```python
from build123d import *

# Parameters (mm, degrees)
SKETCH002_R           = 15
SKETCH002_R_2         = 13.55
PAD002_DEPTH          = 3
PAD002_DEPTH_BACK     = 1.4
CHAMFER001_SIZE       = 1
CHAMFER002_SIZE       = 0.6
SKETCH003_R           = 13.55
PAD003_DEPTH          = 1
SKETCH004_W           = 1.1
SKETCH004_H           = 2.4
POCKET_DEPTH          = 0.8
SKETCH005_R           = 13.55
SKETCH005_R_2         = 12
PAD005_DEPTH          = 2
PAD006_DEPTH          = 2
POLARPATTERN001_COUNT = 4
SKETCH007_R           = 9.5
POCKET001_DEPTH       = 0.6
SKETCH008_R           = 1.3
POCKET002_DEPTH       = 7


with BuildPart() as part:
    # Sketch002 → Pad002 (new body, two sides)
    with BuildSketch(Plane.XY) as pad002_sk:
        Circle(SKETCH002_R)
        Circle(SKETCH002_R_2, mode=Mode.SUBTRACT)
    extrude(amount=-PAD002_DEPTH)
    extrude(pad002_sk.sketch, amount=PAD002_DEPTH_BACK)

    # Chamfer001
    chamfer001_edges = [part.edges().sort_by_distance(p)[0] for p in [
        (-15, 0, 1.4),
    ]]
    chamfer(chamfer001_edges, length=CHAMFER001_SIZE)

    # Chamfer002
    chamfer002_edges = [part.edges().sort_by_distance(p)[0] for p in [
        (-15, 0, -3),
    ]]
    chamfer(chamfer002_edges, length=CHAMFER002_SIZE)

    # Sketch003 → Pad003 (join)
    with BuildSketch(Plane.XY.offset(-3)):
        Circle(SKETCH003_R)
    extrude(amount=PAD003_DEPTH)

    # Sketch004 → Pocket (cut)
    with BuildSketch(Plane.XY):
        with Locations((13.5, 0)):
            Rectangle(SKETCH004_W, SKETCH004_H)
    pocket = extrude(amount=POCKET_DEPTH, mode=Mode.SUBTRACT)

    # Sketch005 → Pad005 (join)
    with BuildSketch(Plane.XY):
        Circle(SKETCH005_R)
        Circle(SKETCH005_R_2, mode=Mode.SUBTRACT)
    extrude(amount=-PAD005_DEPTH)

    # Sketch006 → Pad006 (join)
    with BuildSketch(Plane.XY):
        with BuildLine():
            ThreePointArc((12.310097, -2.170602), (12.5, 0), (12.310097, 2.170602))
            Line((7.878462, 1.389185), (12.310097, 2.170602))
            ThreePointArc((7.878462, -1.389185), (8, 0), (7.878462, 1.389185))
            Line((7.878462, -1.389185), (12.310097, -2.170602))
        make_face()
    pad006 = extrude(amount=-PAD006_DEPTH)

    # PolarPattern001: Pocket, Pad006 ×4 about axis
    polarpattern001_axis = Axis((0, 0, 0), (0, 0, 1))
    for i in range(1, POLARPATTERN001_COUNT):
        add(pocket.rotate(polarpattern001_axis, i * 360 / POLARPATTERN001_COUNT), mode=Mode.SUBTRACT)
        add(pad006.rotate(polarpattern001_axis, i * 360 / POLARPATTERN001_COUNT))

    # Sketch007 → Pocket001 (cut)
    with BuildSketch(Plane.XY):
        Circle(SKETCH007_R)
    extrude(amount=-POCKET001_DEPTH, mode=Mode.SUBTRACT)

    # Sketch008 → Pocket002 (cut)
    with BuildSketch(Plane(origin=(11, -11, 0), x_dir=(0.707107, 0.707107, 0), z_dir=(0.707107, -0.707107, 0))):
        with Locations((0, -1.3)):
            Circle(SKETCH008_R)
    extrude(amount=-POCKET002_DEPTH, mode=Mode.SUBTRACT)


solid = part.part
```
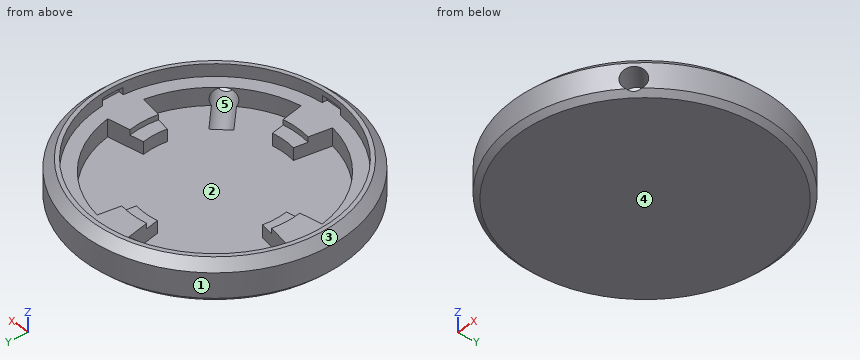
The listing builds one solid part. Answer for the finished solid, in the listing's coordinates (mm). Face numbers are marked on the shaded views. A direction names the side the tool comes from. Round coordinates to 2 decimals unless told otherwise and drop trailing zeros. Loops run counter-clockwise (first coordinate to the right, second up) from the corner with the lowest first, then second, coordinate; pieces in that order, holes last. Notation, with made-up numbers: (42.25, 29.25) - (96.25, 29.25) arc R27 ccw to (96.25, 48.25) - close; hole circle Ø5 at (60, -38). An arc over 180 degrees is marked (long way). Return JSON: item names as keys, results as strings. Group by question number.
1. The part is cut by section C-C on z = -1.65. Determine the outline of the cut face in (x, y), then the cut area to 3 significant figures.
2. Consider probe 1 along Y at (x, z) = (0, 0.4); probe 2 along X at (y, z) = (9, -1.9); probe 3 along Y at (x, z) = (-8.5, -1.3). Determine where each line is inside the solid, lowest interval first.
3. Each of these flat-tipped pins is pushed along its axis until it touches: P1, Ø1.3, axis at x = 0, y = 9, coming from the +Z side; P2, Ø0.6, axis at x = 14, z = 0.5, coming from the -Y side; P3, Ø1.3, axis at x = -1, y = -8.5, coming from the +Z side. Where does it stop, or does it pass through?
4. Which of the six approach directions +Z, -Z, +X, -X, +Y, -Y give full straight-line access (tool end or side, diameter ignored) to the marked faces 1 and 2?
5. The part is cut by section A-A on x = 0. Determine the outline of the cut face in (y, z).
6. The mould has two halves that part along Y. Classify the marked faces 3, 4 and 5: pulls with the +Y half, pulls with the -Y half, needs draft (parallel to the pull), parting line crosses it, or undercut.
Resolved:
{
 "1": {"outline": "(-11.82, -2.08) - (-7.88, -1.39) arc R8 cw to (-7.88, 1.39) - (-11.82, 2.08) arc R12 cw to (-2.08, 11.82) - (-1.39, 7.88) arc R8 cw to (1.39, 7.88) - (2.08, 11.82) arc R12 cw to (11.82, 2.08) - (7.88, 1.39) arc R8 cw to (7.88, -1.39) - (11.82, -2.08) arc R12 cw to (9.32, -7.55) - (11.45, -9.68) arc R15 ccw (long way) to (9.68, -11.45) - (7.55, -9.32) arc R12 cw to (2.08, -11.82) - (1.39, -7.88) arc R8 cw to (-1.39, -7.88) - (-2.08, -11.82) arc R12 cw to start", "area": "303 mm²"},
 "2": {"probe 1": "y = -15 to -14.05, 14.05 to 15", "probe 2": "x = -12 to -7.94, -1.59 to 1.59, 7.94 to 12", "probe 3": "y = -12.36 to -8.47, -1.5 to 1.5, 8.47 to 12.36"},
 "3": {"P1": "stops at z = 0", "P2": "stops at y = -6.07", "P3": "stops at z = -0.6"},
 "4": {"face 1": "+Z, -Z", "face 2": "+Z"},
 "5": {"outline": "(-15, -2.4) - (-14.4, -3) - (14.4, -3) - (15, -2.4) - (15, 0.4) - (14, 1.4) - (13.55, 1.4) - (13.55, 0.8) - (14.05, 0.8) - (14.05, 0) - (9.5, 0) - (9.5, -0.6) - (8, -0.6) - (8, -2) - (-8, -2) - (-8, -0.6) - (-9.5, -0.6) - (-9.5, 0) - (-14.05, 0) - (-14.05, 0.8) - (-13.55, 0.8) - (-13.55, 1.4) - (-14, 1.4) - (-15, 0.4) - close"},
 "6": {"face 3": "parting line crosses it", "face 4": "needs draft", "face 5": "undercut"}
}
